Build history of the part. All positions in model axes, mm. A direction names the side the tool comes from. Coordinates: 2 decimals unless noted, no trailing zeros. Loops run counter-clockwise (first coordinate to the right, second up) from the corner with the lowest first, then second, coordinate; pieces in that order, holes last. Notation, with made-up numbers: (33, 29) -> (83, 29) arc R29 cw to (83, 53) -> close; hole circle Ø2 at (70.25, 69.5). An arc over 180 degrees is marked (long way). One line per item, written item: value. Start each with the question number.
```python
from build123d import *

# Parameters (mm, degrees)
BOSS_EXTRUDE1_DEPTH       = 25.4
SKETCH3_R                 = 6.35
CUT_EXTRUDE1_DEPTH        = 39.1
F_4_CLEARANCE_HOLE1_D     = 3.2639
F_4_CLEARANCE_HOLE1_DEPTH = 3.175
F_4_CLEARANCE_HOLE1_TIP   = 0.980574487


with BuildPart() as part:
    # Sketch1 → Boss-Extrude1 (new, symmetric)
    with BuildSketch(Plane.XY):
        Polygon((0, 0), (12.7, 0), (12.7, 1.5875), (1.5875, 1.5875), (1.5875, 25.4), (0, 25.4), align=None)
    extrude(amount=BOSS_EXTRUDE1_DEPTH, both=True)

    # Sketch3 → Cut-Extrude1 (cut, through all)
    with BuildSketch(Plane.ZY):
        with Locations((11.1125, 17.78)):
            Circle(SKETCH3_R)
        with Locations((-11.1125, 17.78)):
            Circle(SKETCH3_R)
    extrude(amount=-CUT_EXTRUDE1_DEPTH, mode=Mode.SUBTRACT)

    # #4 Clearance Hole1
    with Locations(Plane(origin=(0, 1.5875, 0), x_dir=(1, 0, 0), z_dir=(0, 1, 0))):
        with Locations((7.9375, 19.05), (7.9375, -19.05)):
            Hole(F_4_CLEARANCE_HOLE1_D / 2, depth=F_4_CLEARANCE_HOLE1_DEPTH)
            with Locations((0, 0, -(F_4_CLEARANCE_HOLE1_DEPTH + F_4_CLEARANCE_HOLE1_TIP / 2))):  # 118° drill point
                Cone(0, F_4_CLEARANCE_HOLE1_D / 2, F_4_CLEARANCE_HOLE1_TIP, mode=Mode.SUBTRACT)


solid = part.part
```
Item 1: Drop flat-ended pins along their axis: pin 1 Ø14.5 at (y, z) = (17.78, 11.11) entering from +X; pin 2 Ø5.5 at (x, z) = (5, -3) entering from +Y; pin 3 Ø3 at (x, z) = (7.94, 19.05) entering from -Y. Give the stop position or say it passes through.
Item 2: Tool access for faces 4 (the face through (1.588, 11, 0)), 5 (the face through (0, 13, 0)): list every direction of +Z, -Z, +X, -X, +Y, -Y with a clear straight run to the whole face (end or side of a thin tool).
Item 3: Band-saw the part on B-B, the plane y = 17.78. List the corners of the cut face in (x, z), and give its area (3 significant figures).
Item 4: Band-saw the part on A-A, the plane z = -19.05. List the corners of the cut face in (x, y), and give its area (3 significant figures).
Item 5: Probe probe 1 along X at (y, z) = (1.25, -19.05); probe 2 along X at (y, z) = (23, -16). List the from-to ranges inside material, lowest first.
Item 6: Two-plate mould, pull along Y, no slides. Class faces 1 (the face through (6, 0, 0)), 2 (the face through (0.783, 24.076, -11.939)), 3 (the face through (1, 9, 25.4)): +Y half, -Y half, draft (parallel to the pull), parting line (faces both ways), or undercut.
Item 7: Band-saw the part on C-C, the plane x = 7.25. List the corners of the cut face in (y, z), and give its area (3 significant figures).
Item 8: Band-saw the part on D-D, the plane z = 8.5. List the corners of the cut face in (x, y).
Worked out:
1. pin 1: stops at x = 1.59
1. pin 2: stops at y = 1.59
1. pin 3: passes through
2. face 4: +Z, -Z, +X, +Y
2. face 5: +Z, -Z, -X, +Y, -Y
3. outline: (0, -25.4) -> (1.59, -25.4) -> (1.59, -17.46) -> (0, -17.46) -> close; (0, -4.76) -> (1.59, -4.76) -> (1.59, 4.76) -> (0, 4.76) -> close; (0, 17.46) -> (1.59, 17.46) -> (1.59, 25.4) -> (0, 25.4) -> close
3. area: 40.3 mm²
4. outline: (0, 0) -> (6.31, 0) -> (6.31, 1.59) -> (1.59, 1.59) -> (1.59, 25.4) -> (0, 25.4) -> close; (9.57, 0) -> (12.7, 0) -> (12.7, 1.59) -> (9.57, 1.59) -> close
4. area: 52.8 mm²
5. probe 1: x = 0 to 6.31, 9.57 to 12.7
5. probe 2: x = 0 to 1.59
6. face 1: -Y half
6. face 2: undercut
6. face 3: draft
7. outline: (0, -25.4) -> (1.59, -25.4) -> (1.59, -20.53) -> (0, -20.53) -> close; (0, -17.57) -> (1.59, -17.57) -> (1.59, 17.57) -> (0, 17.57) -> close; (0, 20.53) -> (1.59, 20.53) -> (1.59, 25.4) -> (0, 25.4) -> close
7. area: 71.2 mm²
8. outline: (0, 0) -> (12.7, 0) -> (12.7, 1.59) -> (1.59, 1.59) -> (1.59, 11.99) -> (0, 11.99) -> close; (0, 23.57) -> (1.59, 23.57) -> (1.59, 25.4) -> (0, 25.4) -> close
